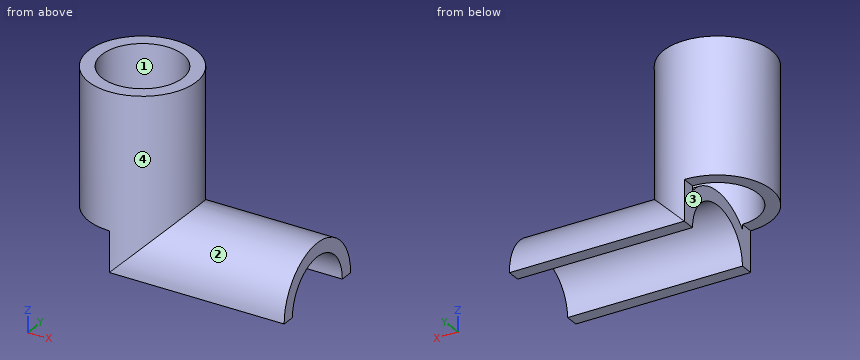
from build123d import *

# Parameters (mm, degrees)
F0_R     = 10.16
F0_R_2   = 7.62
F1_DEPTH = 25.4
F3_DEPTH = 25.4
F5_DEPTH = 46.736
F7_DEPTH = 7.62
F8_DEPTH = 7.62
F9_DEPTH = 7.62


with BuildPart() as f1:
    # F0 (on Top) → F1 (new body)
    with BuildSketch(Plane.XY):
        Circle(F0_R)
        Circle(F0_R_2, mode=Mode.SUBTRACT)
    extrude(amount=F1_DEPTH)

    # F2 (on Right) → F3 (join)
    with BuildSketch(Plane.YZ):
        with BuildLine():
            Line((-10.16, 0), (-7.5868873905, 0))
            ThreePointArc((-7.5868873905, 0), (0, 7.5868873905), (7.5868873905, 0))
            Line((7.5868873905, 0), (10.16, 0))
            ThreePointArc((10.16, 0), (0, 10.16), (-10.16, 0))
        make_face()
    extrude(amount=F3_DEPTH)

    # F4 (on Right) → F5 (cut)
    with BuildSketch(Plane.YZ):
        with BuildLine():
            ThreePointArc((7.62, 0), (0, 7.62), (-7.62, 0))
            Line((-7.62, 0), (7.62, 0))
        make_face()
    extrude(amount=F5_DEPTH, mode=Mode.SUBTRACT)

    # F6 (on face) → F7 (cut)
    with BuildSketch(Plane(origin=(0, 0, 0), x_dir=(1, 0, 0), z_dir=(0, 0, -1))):
        with BuildLine():
            Line((0, 7.62), (0, 10.16))
            ThreePointArc((0, 10.16), (-10.16, 0), (0, -10.16))
            Line((0, -10.16), (0, -7.62))
            ThreePointArc((0, -7.62), (-7.62, 0), (0, 7.62))
        make_face()
    extrude(amount=-F7_DEPTH, mode=Mode.SUBTRACT)

    # F8 (add): a face of the model
    f8_faces = [f1.faces().sort_by_distance(p)[0] for p in [
        (-9.8726318041, 0, 25.4),
    ]]
    extrude(f8_faces, amount=F8_DEPTH)

    # F9 (add): a face of the model
    f9_faces = [f1.faces().sort_by_distance(p)[0] for p in [
        (25.4, 0, 7.8471845065),
    ]]
    extrude(f9_faces, amount=F9_DEPTH)


solid = f1.part
CAD build for the part. Positions are in the model's coordinates, mm. Face numbers are marked on the shaded views. Give positions to 0.01 mm unless a question says otherwise; leave off trailing zeros. Loops run counter-clockwise (first coordinate to the right, second up) from the corner with the lowest first, then second, coordinate; pieces in that order, holes last. Notation, with made-up numbers: M 39.25,-34 L 84.25,-34 A18 ccw 84.25,-13 Z; hole C -19,-35 d9. An arc over 180 degrees is marked long. Write each question's results on one line, items separated by ' | '.
Q1. Flat gauge pins, fed straight in: P1, Ø5, axis at x = 3, z = 28, coming from the +Y side; P2, Ø1, axis at x = 1, z = 17.5, coming from the -Y side; P3, Ø2, axis at y = 5.5, z = 29.5, coming from the -X side. Where does each tip first touch, or does it go through?
Geometry check:
P1: stops at y = 10.15 | P2: stops at y = -10.15 | P3: stops at x = -9.11
Q2. Mould opens along X. For the marked faces 1, 2, 3 and 4 say: pulls with the +X half, pulls with the -X half, needs draft (parallel to the pull), parting line crosses it, or undercut.
Geometry check:
face 1: undercut | face 2: needs draft | face 3: undercut | face 4: parting line crosses it
Q3. Band-saw the part on A-A on y = 0. Write the cut outline in (x, z).
Geometry check:
outline: M -10.16,7.62 L -7.62,7.62 L -7.62,33.02 L -10.16,33.02 Z; M 0,7.62 L 33.02,7.62 L 33.02,10.16 L 10.16,10.16 L 10.16,33.02 L 7.62,33.02 L 7.62,10.16 L 0,10.16 Z
Q4. Band-saw the part on B-B on x = -5. Write the cut outline in (y, z).
Geometry check:
outline: M -8.84,7.62 L -5.75,7.62 L -5.75,33.02 L -8.84,33.02 Z; M 5.75,7.62 L 8.84,7.62 L 8.84,33.02 L 5.75,33.02 Z
Q5. Band-saw the part on C-C on z = 25. Write the cut outline in (x, y).
Geometry check:
outline: C 0,0 d20.32; hole C 0,0 d15.24
Q6. Band-saw the part on D-D on y = -6. Write the cut outline in (x, z).
Geometry check:
outline: M -8.2,7.62 L -4.7,7.62 L -4.7,33.02 L -8.2,33.02 Z; M 0,4.7 L 33.02,4.7 L 33.02,8.2 L 8.2,8.2 L 8.2,33.02 L 4.7,33.02 L 4.7,8.2 L 0,8.2 Z
Q7. Probe probe 1 along Y at (x, z) = (0, 12); probe 2 along Y at (x, z) = (1.5, 11). List the from-to ranges inside material, lowest first.
Geometry check:
probe 1: y = -10.16 to -7.62, 7.62 to 10.16 | probe 2: y = -10.05 to -7.47, 7.47 to 10.05
